```python
from build123d import *

# Parameters (mm, degrees)
SKETCH1_W           = 250
SKETCH1_H           = 46.98
BOSS_EXTRUDE1_DEPTH = 3
SKETCH2_W           = 3
SKETCH2_H           = 20
CUT_EXTRUDE1_DEPTH  = 255.393632782
SKETCH3_W           = 60
SKETCH3_H           = 3
CUT_EXTRUDE2_DEPTH  = 255.393632782
CUT_EXTRUDE3_REACH  = 256.394
SKETCH4_W           = 90
SKETCH4_H           = 20
SKETCH6_W           = 20
SKETCH6_H           = 3
SKETCH6_W_2         = 30
CUT_EXTRUDE5_DEPTH  = 10


with BuildPart() as part:
    # Sketch1 → Boss-Extrude1 (new body)
    with BuildSketch(Plane.XY):
        with Locations((125, 23.49)):
            Rectangle(SKETCH1_W, SKETCH1_H)
    extrude(amount=BOSS_EXTRUDE1_DEPTH)

    # Sketch2 → Cut-Extrude1 (cut, through all)
    with BuildSketch(Plane.XY.offset(3)):
        with Locations((248.5, 26.98)):
            Rectangle(SKETCH2_W, SKETCH2_H)
        with Locations((1.5, 26.98)):
            Rectangle(SKETCH2_W, SKETCH2_H)
    extrude(amount=-CUT_EXTRUDE1_DEPTH, mode=Mode.SUBTRACT)

    # Sketch3 → Cut-Extrude2 (cut, through all)
    with BuildSketch(Plane.XY.offset(3)):
        with Locations((50, 45.48)):
            Rectangle(SKETCH3_W, SKETCH3_H)
        with Locations((200, 45.48)):
            Rectangle(SKETCH3_W, SKETCH3_H)
    extrude(amount=-CUT_EXTRUDE2_DEPTH, mode=Mode.SUBTRACT)

    # Sketch4 → Cut-Extrude3 (cut, up to next)
    with BuildSketch(Plane(origin=(0, 0, 0), x_dir=(-1, 0, 0), z_dir=(0, 0, -1)), mode=Mode.PRIVATE) as cut_extrude3_sk1:
        with Locations((-125, 10)):
            Rectangle(SKETCH4_W, SKETCH4_H)
    cut_extrude3_tool1 = extrude(cut_extrude3_sk1.sketch, amount=-CUT_EXTRUDE3_REACH, mode=Mode.PRIVATE) & part.part
    add(cut_extrude3_tool1.solids().sort_by_distance((125, 10, 0))[0], mode=Mode.SUBTRACT)

    # Sketch6 → Cut-Extrude5 (cut)
    with BuildSketch(Plane.XY.offset(3)):
        with Locations((10, 1.5)):
            Rectangle(SKETCH6_W, SKETCH6_H)
        with Locations((65, 1.5)):
            Rectangle(SKETCH6_W_2, SKETCH6_H)
        with Locations((240, 1.5)):
            Rectangle(SKETCH6_W, SKETCH6_H)
        with Locations((185, 1.5)):
            Rectangle(SKETCH6_W_2, SKETCH6_H)
    extrude(amount=-CUT_EXTRUDE5_DEPTH, mode=Mode.SUBTRACT)


solid = part.part
```
The listing builds one solid part. Answer for the finished solid, in the listing's coordinates (mm). Give positions to 0.01 mm unless a question says otherwise; leave off trailing zeros. Write each loop counter-clockwise with the first axis right and the second up, starting at its lowest first coordinate (ties: lowest second). Pieces come first, ordered by that corner, then holes. Notation, with made-up numbers: (-38.5, 12.5) -> (-3.5, 12.5) arc R12 cw to (-3.5, 32.5) -> close; hole circle Ø5 at (33, 1). An arc over 180 degrees is marked (long way). Use one line per item in the form item = value.
1) Section A-A on y = 11 is taken. Write down the section's boundary in (x, z).
Result:
outline = (0, 0) -> (80, 0) -> (80, 3) -> (0, 3) -> close; (170, 0) -> (250, 0) -> (250, 3) -> (170, 3) -> close
2) Each of these flat-tipped pins is pushed along its axis until it touches: P1, Ø1, axis at x = 208.5, z = 2, coming from the +Y side; P2, Ø1.5, axis at x = 172.5, z = 1.5, coming from the -Y side; P3, Ø1.5, axis at y = 1.5, z = 1, coming from the +X side. Where does it stop, or does it pass through?
Result:
P1 = 43.98
P2 = 3
P3 = 230
3) Section D-D on x = 180 is taken. Write down the section's boundary in (y, z), plus the area to 3 significant figures.
Result:
outline = (3, 0) -> (43.98, 0) -> (43.98, 3) -> (3, 3) -> close
area = 123 mm²
4) Section C-C on y = 33.5 is taken. Write down the section's boundary in (x, z).
Result:
outline = (3, 0) -> (247, 0) -> (247, 3) -> (3, 3) -> close
5) Straight lines are drawn through the part: probe 1 along X at (y, z) = (5.5, 1.6); probe 2 along X at (y, z) = (19.5, 2.5); probe 3 along X at (y, z) = (22, 2.2). For each, find the intervals that lie inside material, in ascending order.
Result:
probe_1 = 0 to 80, 170 to 250
probe_2 = 3 to 80, 170 to 247
probe_3 = 3 to 247
